```python
from build123d import *


with BuildPart() as part:
    # Sketch → Revolution (revolve)
    with BuildSketch(Plane.XZ):
        Polygon((4, 0), (4, 3.5), (5.5, 3.5), (5.5, 3), (6, 3), (6, 3.5), (8, 3.5), (8.925, 3), (9.85, 3.5), (11, 3.5), (11, 0), align=None)
    revolution = revolve(axis=Axis((0, 0, 0), (0, 0, 1)))

    # Mirrored: Revolution across XY
    add(revolution.mirror(Plane.XY))


solid = part.part
```
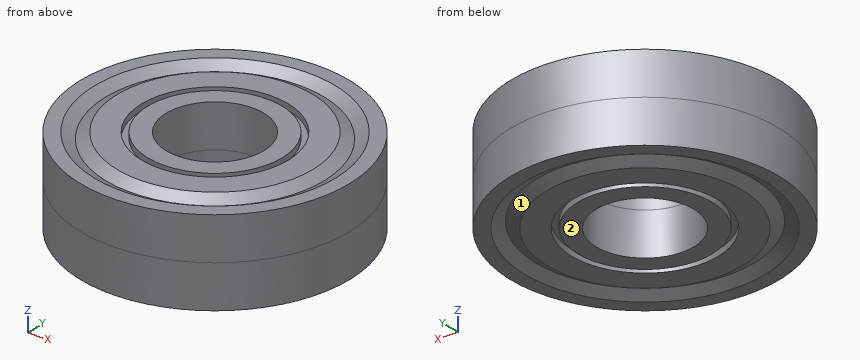
Check sheet for the modelled part. Datum: model origin and axes. Units: mm. Face numbers are marked on the shaded views. Round coordinates to 2 decimals unless told otherwise and drop trailing zeros. Loops run counter-clockwise (first coordinate to the right, second up) from the corner with the lowest first, then second, coordinate; pieces in that order, holes last. Notation, with made-up numbers: (41, 54) - (77, 54) arc R18 cw to (77, 82) - close; hole circle Ø5 at (77.5, -27.5). An arc over 180 degrees is marked (long way). Answer as a JSON object with one key per item and string values. Group by question number.
Q1. Gauge pin test, flat ends, axial feed: P1, Ø8, axis at x = -0.5, y = -8.5, coming from the +Z side; P2, Ø1.5, axis at x = -5, z = 1, coming from the -Y side; P3, Ø6.5, axis at x = 0, y = 0, coming from the -Z side; P4, Ø1.5, axis at y = 1, z = -1, coming from the +X side. Record the tip position at first contact, or that the pin passes through.
Q2. Mould release check, pull along Y, two halves, no side actions. Record for the marked faces 1 and 2: released by +Y, released by -Y, zero draft, split by the parting line, or undercut.
Q3. Scan lines: line 1 along Y through (x, z) = (0, 3.15); line 2 along Y through (x, z) = (0, -1.75); line 3 along X through (y, z) = (-4.75, 3.25). Record each from-to range of solid material in increasing order. Write a range as [from, to].
Q4. Sectioned sample at A-A, the plane z = -0.5. Enter the section's corners in (x, y).
Solution:
{
 "1": {"P1": "stops at z = 3.5", "P2": "stops at y = -10.15", "P3": "passes through", "P4": "stops at x = 11"},
 "2": {"face 1": "undercut", "face 2": "zero draft"},
 "3": {"line 1": "y = [-11, -9.2], [-8.65, -6], [-5.5, -4], [4, 5.5], [6, 8.65], [9.2, 11]", "line 2": "y = [-11, -4], [4, 11]", "line 3": "x = [-9.92, -8.1], [-7, -3.67], [-2.77, 2.77], [3.67, 7], [8.1, 9.92]"},
 "4": {"outline": "circle Ø22 at (0, 0); hole circle Ø8 at (0, 0)"}
}
